Drawing for the job (mm, zero at the part's lowest x, y, z). A direction names the side the tool comes from. Give positions to 0.01 mm unless a question says otherwise; leave off trailing zeros. Loops run counter-clockwise (first coordinate to the right, second up) from the corner with the lowest first, then second, coordinate; pieces in that order, holes last. Notation, with made-up numbers: (58, 89) -> (68, 89) arc R13 cw to (68, 112) -> close; hole circle Ø11 at (58, -12.75). An arc over 180 degrees is marked (long way). Answer in a Markdown table with one row per item. Add a question column.
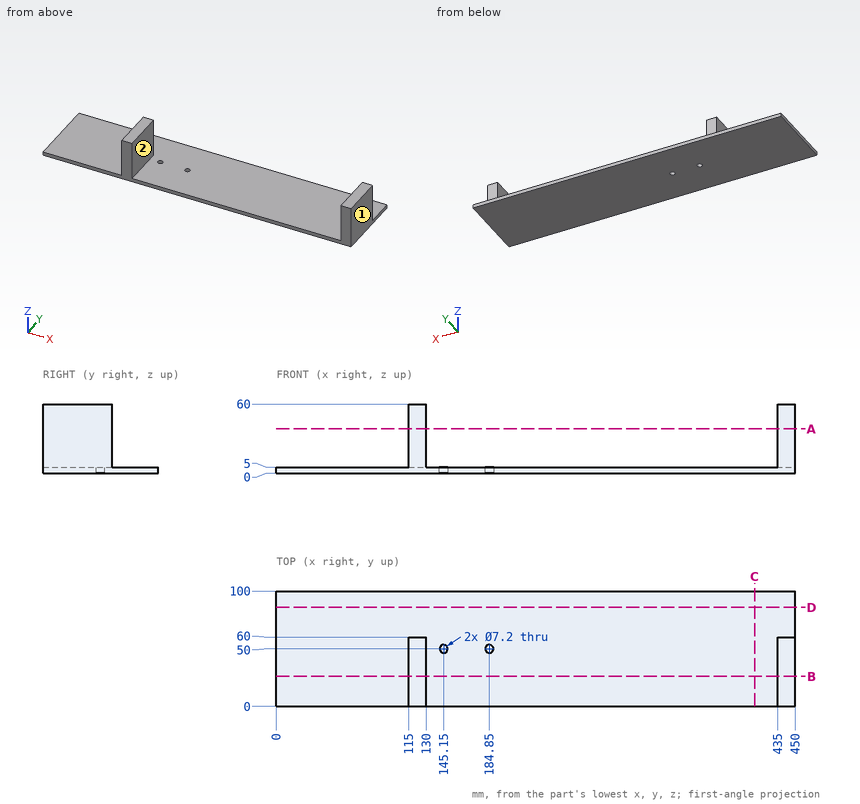
(1) Flat gauge pins, fed straight in: pin 1 Ø3 at (x, y) = (322.5, 82.5) entering from +Z; pin 2 Ø6.5 at (x, y) = (184.85, 50) entering from +Z; pin 3 Ø12 at (x, z) = (123, 39) entering from +Y; pin 4 Ø4 at (x, y) = (186, 32.5) entering from -Z. Where does each tip first touch, or does it go through?
(2) 3-axis set-ups, long thin cutter, end or side, ignore diameter. For the marked faces 1 and 2: which of +Z, -Z, +X, -X, +Y, -Y reach the whole face in a straight line?
(3) Saw through at B-B, the plane y = 26. List the corners of the cut face in (x, z), then the cut area to 3 significant figures.
(4) Wall check: line 1 along X through (y, z) = (5.5, 20.5); line 2 along Y through (x, z) = (145.15, 2.5); line 3 along Z through (x, y) = (339, 24.5). Give the ranges that are in metal, low to high. Write a range as from..to.
(5) Saw through at D-D, the plane y = 86. List the corners of the cut face in (x, z).
(6) Saw through at C-C, the plane x = 415. List the corners of the cut face in (y, z).
(7) Saw through at A-A, the plane z = 38.5. List the corners of the cut face in (x, y), then the cut area to 3 significant figures.
Worked answers:
| question | item | result |
|---|---|---|
| 1 | pin 1 | z = 5 |
| 1 | pin 2 | through |
| 1 | pin 3 | y = 60 |
| 1 | pin 4 | z = 0 |
| 2 | face 1 | +Z, -Z, +X, +Y, -Y |
| 2 | face 2 | +Z, +Y, -Y |
| 3 | outline | (0, 0) -> (450, 0) -> (450, 60) -> (435, 60) -> (435, 5) -> (130, 5) -> (130, 60) -> (115, 60) -> (115, 5) -> (0, 5) -> close |
| 3 | area | 3,900 mm^2 |
| 4 | line 1 | 115..130, 435..450 |
| 4 | line 2 | 0..46.4, 53.6..100 |
| 4 | line 3 | 0..5 |
| 5 | outline | (0, 0) -> (450, 0) -> (450, 5) -> (0, 5) -> close |
| 6 | outline | (0, 0) -> (100, 0) -> (100, 5) -> (0, 5) -> close |
| 7 | outline | (115, 0) -> (130, 0) -> (130, 60) -> (115, 60) -> close; (435, 0) -> (450, 0) -> (450, 60) -> (435, 60) -> close |
| 7 | area | 1,800 mm^2 |
